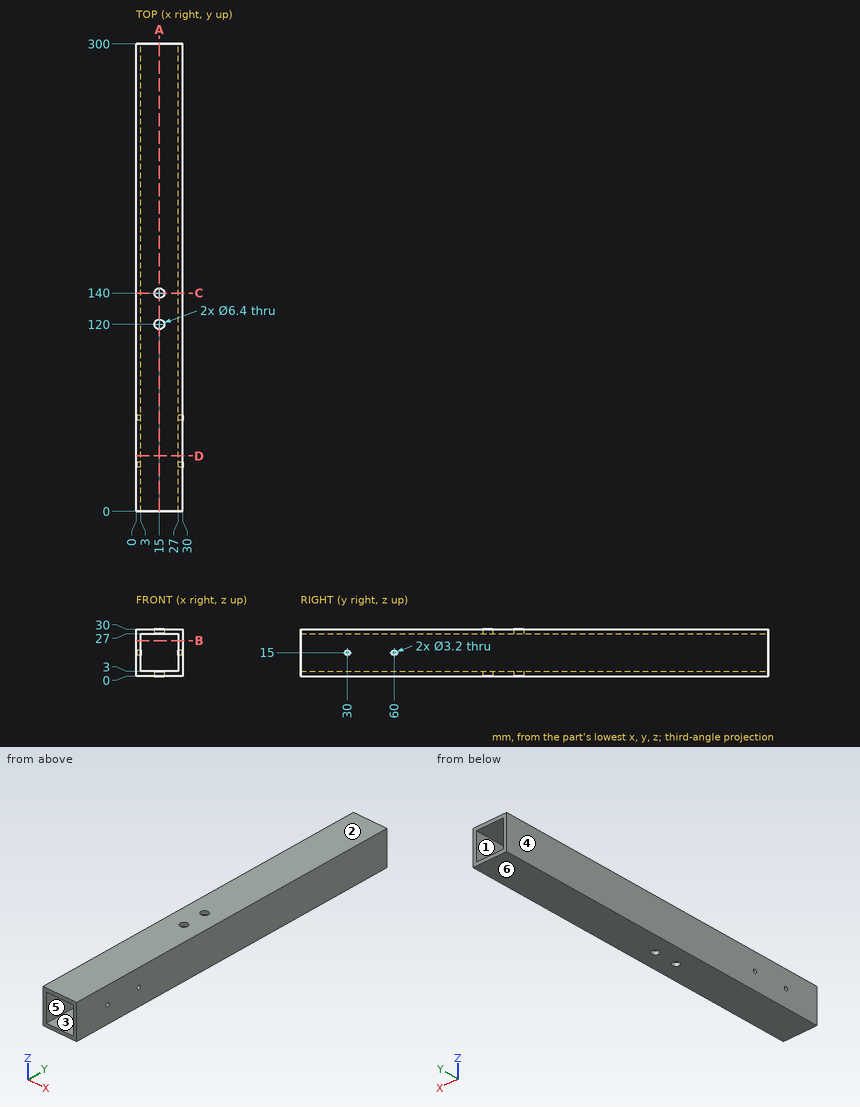
Here's the drawing with two shaded views (mm, measured from the low corner). I have some questions. A direction names the side the tool comes from. Coordinates: 2 decimals unless noted, no trailing zeros. Loops run counter-clockwise (first coordinate to the right, second up) from the corner with the lowest first, then second, coordinate; pieces in that order, holes last.
Item 1: If we mould it in two halves opening along X, with no side actions, what happens to the marked faces 1, 2, 3 and 4? For each: released by +X, released by -X, zero draft, split by the parting line, or undercut.
Answers below:
face 1: undercut
face 2: zero draft
face 3: undercut
face 4: released by -X
Item 2: Suppose I cut it at C-C (y = 140). Please give me the cut outline in (x, z), then the cut area to 3 significant figures.
Answers below:
outline: (0, 0) - (11.8, 0) - (11.8, 3) - (3, 3) - (3, 27) - (11.8, 27) - (11.8, 30) - (0, 30) - close; (18.2, 0) - (30, 0) - (30, 30) - (18.2, 30) - (18.2, 27) - (27, 27) - (27, 3) - (18.2, 3) - close
area: 286 mm2
Item 3: I'm going to push a flat-ended pin straight in: pin 1 (5 mm diameter, centred on x = 15, y = 140, fed in from +Z). Where does the tip first touch, or does it pass through?
Answers below:
pin 1: passes through
Item 4: Which directions (+Z, -Z, +X, -X, +Y, -Y) give clear straight access to the entire face, cutting with the end or side of a thin tool? Please do the marked faces 5 and 6.
Answers below:
face 5: +Y, -Y
face 6: -Z, +X, -X, +Y, -Y
Item 5: Suppose I cut it at B-B (z = 22.75). Please give me the cut outline in (x, y), then the cut area to 3 significant figures.
Answers below:
outline: (0, 0) - (3, 0) - (3, 300) - (0, 300) - close; (27, 0) - (30, 0) - (30, 300) - (27, 300) - close
area: 1,800 mm2
Item 6: Suppose I cut it at A-A (x = 15). Please give me the cut outline in (y, z), then the cut area to 3 significant figures.
Answers below:
outline: (0, 0) - (116.8, 0) - (116.8, 3) - (0, 3) - close; (0, 27) - (116.8, 27) - (116.8, 30) - (0, 30) - close; (123.2, 0) - (136.8, 0) - (136.8, 3) - (123.2, 3) - close; (123.2, 27) - (136.8, 27) - (136.8, 30) - (123.2, 30) - close; (143.2, 0) - (300, 0) - (300, 3) - (143.2, 3) - close; (143.2, 27) - (300, 27) - (300, 30) - (143.2, 30) - close
area: 1,720 mm2
Item 7: Suppose I cut it at D-D (y = 35.5). Please give me the cut outline in (x, z).
Answers below:
outline: (0, 0) - (30, 0) - (30, 30) - (0, 30) - close; hole (3, 3) - (27, 3) - (27, 27) - (3, 27) - close
Item 8: Please list where these lines run through material, in increasing order: L1, parallel to Y at x = 15, z = 28.25; L2, parallel to Y at x = 28.4, z = 15; L3, parallel to Z at x = 12.5, y = 50.
Answers below:
L1: y = 0 to 116.8, 123.2 to 136.8, 143.2 to 300
L2: y = 0 to 28.4, 31.6 to 58.4, 61.6 to 300
L3: z = 0 to 3, 27 to 30
